Could you check a few things on this model? Use its own coordinates, in mm. A direction names the side the tool comes from. Give positions to 0.01 mm unless a question says otherwise; leave off trailing zeros. Loops run counter-clockwise (first coordinate to the right, second up) from the corner with the lowest first, then second, coordinate; pieces in that order, holes last. Notation, with made-up numbers: M 34.25,-22.5 L 50.25,-22.5 A21 cw 50.25,16.5 Z; hole C -21,-26.5 d11. An arc over 180 degrees is marked long. Answer in a Markdown table with one row per item. Add a question column.
1. I'm going to push flat-ended pins straight in: pin 1 Ø8 at (y, z) = (41, 9) entering from +X; pin 2 Ø1 at (x, z) = (0.5, 10) entering from +Y; pin 3 Ø1 at (x, z) = (7, 17) entering from +Y; pin 4 Ø6.5 at (x, y) = (6, 50) entering from -Z. Where does each tip first touch, or does it pass through?
2. If we section it at B-B on z = 0: List the corners of the cut face in (x, y) for me, then the cut area to 3 significant figures.
3. If we section it at A-A on x = 6: List the corners of the cut face in (y, z) for me, then the cut area to 3 significant figures.
4. I need wall thicknesses on line 1 along Z through (x, y) = (1.75, 53); line 2 along Y through (x, z) = (5.75, -22); line 3 along X through (y, z) = (50, -1.25). Which ranges of each line are inside material? Lowest first, please. Write a range as from..to.
5. Thinking about a two-plate mould opening in Z: for faces 1 (the flat face through (1, 42.455, 10)), 2 (the flat face through (10.1, 49.1, -15)), 3 (the flat face through (1, 0, 0)), 4 (the cylindrical face through (0.986, 6.014, 19.297)), which applies, released by +Z, released by -Z, zero draft, split by the parting line, or undercut?
6. Which directions (+Z, -Z, +X, -X, +Y, -Y) give clear straight access to the entire face, cutting with the end or side of a thin tool? Please do faces 5 (the flat face through (3.52, 45.64, 0.07)), 6 (the flat face through (0, 25, 0)), 7 (the flat face through (1, 42.455, -10)).
7. If we section it at C-C on y = 4: List the corners of the cut face in (x, z) for me, then the cut area to 3 significant figures.
```python
from build123d import *

# Parameters (mm, degrees)
BOSS_EXTRUDE1_DEPTH                          = 25
SKETCH2_W                                    = 10
SKETCH2_H                                    = 20.590421557
CUT_EXTRUDE1_DEPTH                           = 11
CUT_EXTRUDE1_DEPTH_BACK                      = 3
FILLET1_R                                    = 20
CSK_FOR_M4_COUNTERSUNK_FLAT_HEAD_SCR_2_COUNT = 2
CSK_FOR_M4_COUNTERSUNK_FLAT_HEAD_SCR_2_PITCH = 20.373860658
CSK_FOR_M4_COUNTERSUNK_FLAT_HEAD_SCR_3_COUNT = 2
CSK_FOR_M4_COUNTERSUNK_FLAT_HEAD_SCR_3_PITCH = 20.021215351


with BuildPart() as part:
    # Sketch1 → Boss-Extrude1 (new body, symmetric)
    with BuildSketch(Plane.XY):
        with BuildLine():
            Line((0, 0), (0, 50))
            ThreePointArc((0, 50), (11.186683916, 53.016340491), (3.032769985, 44.785065097))
            Line((3.032769985, 44.785065097), (4.021846657, 46.523376732))
            ThreePointArc((4.021846657, 46.523376732), (9.457789277, 52.01089366), (2, 50))
            Line((2, 50), (2, 0))
            Line((2, 0), (0, 0))
        make_face()
    extrude(amount=BOSS_EXTRUDE1_DEPTH, both=True)

    # Sketch2 → Cut-Extrude1 (cut, two sides)
    with BuildSketch(Plane(origin=(2, 0, 0), x_dir=(0, 0, -1), z_dir=(1, 0, 0))) as cut_extrude1_sk:
        with Locations((-10, 52.749880228)):
            Rectangle(SKETCH2_W, SKETCH2_H)
        with Locations((10, 52.749880228)):
            Rectangle(SKETCH2_W, SKETCH2_H)
    extrude(amount=CUT_EXTRUDE1_DEPTH, mode=Mode.SUBTRACT)
    extrude(cut_extrude1_sk.sketch, amount=-CUT_EXTRUDE1_DEPTH_BACK, mode=Mode.SUBTRACT)

    # Fillet1
    fillet1_edges = [part.edges().sort_by_distance(p)[0] for p in [
        (1, 0, 25),
        (1, 0, -25),
    ]]
    fillet(fillet1_edges, radius=FILLET1_R)

    # Sketch4 → CSK for M4 Countersunk Flat Head Screw1 (revolve, cut)
    with BuildSketch(Plane(origin=(2, 11.587467643, 0), x_dir=(0, 0, -1), z_dir=(0, 1, 0))):
        Polygon((0, 0), (0, 2), (2.25, 2), (2.25, 2.45), (4.7, 0), align=None)
    csk_for_m4_countersunk_flat_head_screw1 = revolve(axis=Axis((8.35, 11.587467643, 0), (-1, 0, 0)), mode=Mode.SUBTRACT)

    # CSK for M4 Countersunk Flat Head Scr 2: CSK for M4 Countersunk Flat Head Screw1 ×2
    with Locations(*[Vector(0, 0.807519759, 0.58984052) * (i * CSK_FOR_M4_COUNTERSUNK_FLAT_HEAD_SCR_2_PITCH) for i in range(1, CSK_FOR_M4_COUNTERSUNK_FLAT_HEAD_SCR_2_COUNT)]):
        add(csk_for_m4_countersunk_flat_head_screw1, mode=Mode.SUBTRACT)

    # CSK for M4 Countersunk Flat Head Scr 3: CSK for M4 Countersunk Flat Head Screw1 ×2
    with Locations(*[Vector(0, 0.77172393, -0.635957683) * (i * CSK_FOR_M4_COUNTERSUNK_FLAT_HEAD_SCR_3_PITCH) for i in range(1, CSK_FOR_M4_COUNTERSUNK_FLAT_HEAD_SCR_3_COUNT)]):
        add(csk_for_m4_countersunk_flat_head_screw1, mode=Mode.SUBTRACT)


solid = part.part
```
Results:
| question | item | result |
|---|---|---|
| 1 | pin 1 | x = 2 |
| 1 | pin 2 | y = 42.45 |
| 1 | pin 3 | y = 55.98 |
| 1 | pin 4 | through |
| 2 | outline | M 0,0 L 2,0 L 2,6.89 L 0,8.89 Z; M 0,14.29 L 2,16.29 L 2,50 A4 cw long 4.02,46.52 L 3.03,44.79 A6 ccw long 0,50 Z |
| 2 | area | 137 mm2 |
| 3 | outline | M 44,-25 L 46,-25 L 46,-15 L 44,-15 Z; M 44,-5 L 46,-5 L 46,5 L 44,5 Z; M 44,15 L 46,15 L 46,25 L 44,25 Z; M 54,-25 L 56,-25 L 56,-15 L 54,-15 Z; M 54,-5 L 56,-5 L 56,5 L 54,5 Z; M 54,15 L 56,15 L 56,25 L 54,25 Z |
| 3 | area | 120 mm2 |
| 4 | line 1 | -25..-15, -5..5, 15..25 |
| 4 | line 2 | 44.01..46.01, 53.99..55.99 |
| 4 | line 3 | 0..2, 10..12 |
| 5 | face 1 | undercut |
| 5 | face 2 | undercut |
| 5 | face 3 | zero draft |
| 5 | face 4 | released by +Z |
| 6 | face 5 | +Z, -Z |
| 6 | face 6 | +Z, -Z, -X, +Y, -Y |
| 6 | face 7 | +X, -X, +Y |
| 7 | outline | M 0,-17 L 2,-17 L 2,17 L 0,17 Z |
| 7 | area | 68.0 mm2 |
